from build123d import *

# Parameters (mm, degrees)
BOSS_EXTRUDE1_DEPTH = 100


with BuildPart() as part:
    # Sketch1 → Boss-Extrude1 (new body)
    with BuildSketch(Plane.XY):
        with BuildLine():
            Line((0, 0), (0, 10))
            add(Edge.make_bspline(
                [(0, 10), (-0.787242099, 34.100733869), (-10.197534483, 50)],
                knots=[0, 0, 0, 1, 1, 1], degree=2))
            Line((-10.197534483, 50), (-18.803177319, 44.906581563))
            add(Edge.make_bspline(
                [(-10, 9.833471065), (-10.030967353, 10.744471696), (-10.114706096, 12.582680835), (-10.361531, 16.119334261), (-10.820269758, 20.371956037), (-11.603430489, 25.176045178), (-12.949670493, 31.196907646), (-14.728828853, 36.634857764), (-16.928703227, 41.544185237), (-18.144309171, 43.793383416), (-18.803177319, 44.906581563)],
                knots=[0.003595485, 0.003595485, 0.003595485, 0.003595485, 0.065870767, 0.12814605, 0.252696614, 0.377247178, 0.501797743, 0.750898871, 0.875449436, 1, 1, 1, 1], degree=3))
            Line((-10, 9.833471065), (-10, 0))
            Line((-10, 0), (-10, -9.833471065))
            add(Edge.make_bspline(
                [(-18.803177319, -44.906581563), (-18.144309171, -43.793383416), (-16.928703227, -41.544185237), (-14.728828853, -36.634857764), (-12.949670493, -31.196907646), (-11.603430489, -25.176045178), (-10.820269758, -20.371956037), (-10.361531, -16.119334261), (-10.114706096, -12.582680835), (-10.030967353, -10.744471696), (-10, -9.833471065)],
                knots=[0.003595485, 0.003595485, 0.003595485, 0.003595485, 0.12814605, 0.252696614, 0.501797743, 0.626348307, 0.750898871, 0.875449436, 0.937724718, 1, 1, 1, 1], degree=3))
            Line((-18.803177319, -44.906581563), (-10.197534483, -50))
            add(Edge.make_bspline(
                [(0, -10), (-0.787242099, -34.100733869), (-10.197534483, -50)],
                knots=[0, 0, 0, 1, 1, 1], degree=2))
            Line((0, -10), (0, 0))
        make_face()
    extrude(amount=BOSS_EXTRUDE1_DEPTH)


solid = part.part
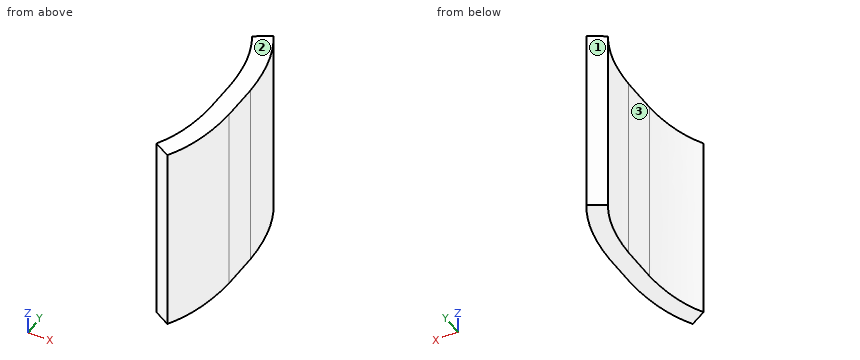
Verification items for the finished model (mm, model axes). Face numbers are marked on the shaded views. Coordinates: 2 decimals unless noted, no trailing zeros. Write each loop counter-clockwise with the first axis right and the second up, starting at its lowest first coordinate (ties: lowest second). Pieces come first, ordered by that corner, then holes. Notation, with made-up numbers: M -35.5,72.5 L -17.5,72.5 A7 cw -17.5,82.5 Z; hole C 27,43 d7. An arc over 180 degrees is marked long. Use a Markdown table: item, result.
Q1. Sectioned sample at A-A, the plane y = 5. Record the boundary of the cut face in (x, z), plus the area to 3 significant figures.
Reply:
| item | result |
|---|---|
| outline | M -10,0 L 0,0 L 0,100 L -10,100 Z |
| area | 1,000 mm² |
Q2. Thickness scan on line 1 (Y direction, x = -16, z = 59.5); line 2 (X direction, y = 0, z = 5.5); line 3 (X direction, y = -36.5, z = 49). Record the ranges inside material, lowest first.
Reply:
| item | result |
|---|---|
| line 1 | y = -46.57 to -39.44, 39.44 to 46.57 |
| line 2 | x = -10 to 0 |
| line 3 | x = -14.8 to -4.22 |
Q3. Draft check along Y on the marked faces 1, 2 and 3. Enter one of: +Y half, -Y half, draft (parallel to the pull), parting line (faces both ways), or undercut.
Reply:
| item | result |
|---|---|
| face 1 | +Y half |
| face 2 | draft |
| face 3 | undercut |
Q4. Go/stop test with flat-tipped pins: P1, Ø8, axis at y = 35.5, z = 86, coming from the -X side; P2, Ø1, axis at x = -9, z = 31.5, coming from the +Y side; P3, Ø21.5, axis at y = -2, z = 61.5, coming from the -X side. Record where each tip stops, or that it passes through.
Reply:
| item | result |
|---|---|
| P1 | stops at x = -16.03 |
| P2 | stops at y = 48.79 |
| P3 | stops at x = -10.14 |
